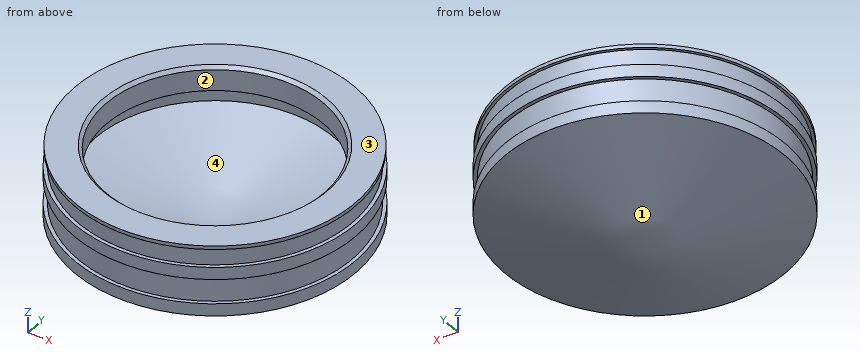
from build123d import *


with BuildPart() as f1:
    # F0 (on Front) → F1 (revolve)
    with BuildSketch(Plane.XZ):
        Polygon((-15.9, 0), (-19.9, 0), (-19.9, -0.5), (-19.5, -0.5), (-19.5, -3), (-20, -3), (-20, -4.75), (-19.5, -4.75), (-19.5, -8.25), (-20, -8.25), (-20, -10), (0, -15.5), (0, -10.595625), (-16.875, -5.955), (-16.875, -3.455), (-15.445, -3.455), (-15.445, -0.455), align=None)
    revolve(axis=Axis((0, 0, -13.047812), (0, 0, 1)))


solid = f1.part
Can you work these out from the model? Positions are in its coordinate system, mm. Face numbers are marked on the shaded views. Round coordinates to 2 decimals unless told otherwise and drop trailing zeros. Write each loop counter-clockwise with the first axis right and the second up, starting at its lowest first coordinate (ties: lowest second). Pieces come first, ordered by that corner, then holes. Notation, with made-up numbers: (-1.5, -8) - (40.5, -8) arc R12 cw to (40.5, 11) - close; hole circle Ø9 at (-1, -25.75). An arc over 180 degrees is marked (long way). Write each question's results on one line, items separated by ' | '. Start each with the question number.
1) Suppose I cut it at C-C (z = -8.75). List the corners of the cut face in (x, y) for me, and give its area (3 significant figures).
2) Suppose I cut it at A-A (z = -1.5). List the corners of the cut face in (x, y) for me (3 decimals), and give its area (3 significant figures).
3) We'd pull the mould along X, two halves only. Please class the marked faces 1, 2, 3 and 4: released by +X, released by -X, zero draft, split by the parting line, or undercut.
4) For pin 1 Ø2 at (y, z) = (-4, -10.5) entering from -X; pin 2 Ø1.5 at (x, y) = (-15.5, -3.5) entering from -Z; pin 3 Ø2 at (x, y) = (-2, -6.5) entering from +Z, each with a flat end and sliding along its axis, tell me the tip position at first contact or that it passes through.
5) Suppose I cut it at B-B (z = -13.75). List the corners of the cut face in (x, y) for me, and give its area (3 significant figures).
6) Please list where these lines run through material, in increasing order: line 1 (Y direction, x = 0, z = -2.4) (3 decimals); line 2 (X direction, y = 0, z = -4.2) (3 decimals).
Here are the results:
1) outline: circle Ø40 at (0, 0); hole circle Ø13.42 at (0, 0) | area: 1,120 mm2
2) outline: circle Ø39 at (0, 0); hole circle Ø30.89 at (0, 0) | area: 445 mm2
3) face 1: split by the parting line | face 2: undercut | face 3: zero draft | face 4: undercut
4) pin 1: stops at x = -19.75 | pin 2: stops at z = -11.34 | pin 3: stops at z = -8.45
5) outline: circle Ø12.73 at (0, 0) | area: 127 mm2
6) line 1: y = -19.5 to -15.445, 15.445 to 19.5 | line 2: x = -20 to -16.875, 16.875 to 20
